from build123d import *

# Parameters (mm, degrees)
SKETCH1_W                = 70
SKETCH1_H                = 70
BOSS_EXTRUDE1_DEPTH      = 500
SKETCH2_W                = 250
SKETCH2_H                = 125
BOSS_EXTRUDE2_DEPTH      = 2
BOSS_EXTRUDE2_DEPTH_BACK = 40


with BuildPart() as part:
    # Sketch1 → Boss-Extrude1 (new body)
    with BuildSketch(Plane.XY):
        Rectangle(SKETCH1_W, SKETCH1_H)
    extrude(amount=BOSS_EXTRUDE1_DEPTH)

    # Sketch2 → Boss-Extrude2 (add, two sides)
    with BuildSketch(Plane(origin=(0, 35, 0), x_dir=(1, 0, 0), z_dir=(0, 1, 0))) as boss_extrude2_sk:
        with Locations((0, -437.5)):
            Rectangle(SKETCH2_W, SKETCH2_H)
    extrude(amount=BOSS_EXTRUDE2_DEPTH)
    extrude(boss_extrude2_sk.sketch, amount=-BOSS_EXTRUDE2_DEPTH_BACK)


solid = part.part
CAD build for the part. Positions are in the model's coordinates, mm. A direction names the side the tool comes from. Coordinates: 2 decimals unless noted, no trailing zeros. Order: outer loops, then holes, each group sorted by start corner. A loop starts at its lowest first (then second) coordinate and runs counter-clockwise, first axis right, second up. Notation, with made-up numbers: (49.5, 7) -> (79.5, 7) arc R18 ccw to (79.5, 21) -> close; hole circle Ø5 at (-19, 72.25). An arc over 180 degrees is marked (long way). Answer in a Markdown table with one row per item.
1) Drill centre lines: line 1 (X direction, y = -25, z = 326); line 2 (Z direction, x = -48.5, y = -1.5); line 3 (Y direction, x = -40.5, z = 452). Where is each one in solid material? Low to high.
Check values:
| item | result |
|---|---|
| line 1 | -35 to 35 |
| line 2 | 375 to 500 |
| line 3 | -5 to 37 |
2) Band-saw the part on A-A (y = 24). List the corners of the cut face in (x, z).
Check values:
| item | result |
|---|---|
| outline | (-125, 375) -> (-35, 375) -> (-35, 0) -> (35, 0) -> (35, 375) -> (125, 375) -> (125, 500) -> (-125, 500) -> close |
3) Flat gauge pins, fed straight in: P1, Ø6, axis at y = -16, z = 415, coming from the +X side; P2, Ø21, axis at y = 10.5, z = 317.5, coming from the -X side; P3, Ø2, axis at x = 52, y = 23, coming from the -Z side. Where does each tip first touch, or does it go through?
Check values:
| item | result |
|---|---|
| P1 | x = 35 |
| P2 | x = -35 |
| P3 | z = 375 |
4) Band-saw the part on B-B (z = 416). List the corners of the cut face in (x, y), and give its area (3 significant figures).
Check values:
| item | result |
|---|---|
| outline | (-125, -5) -> (-35, -5) -> (-35, -35) -> (35, -35) -> (35, -5) -> (125, -5) -> (125, 37) -> (-125, 37) -> close |
| area | 12,600 mm2 |
5) Band-saw the part on C-C (x = 24.5). List the corners of the cut face in (y, z).
Check values:
| item | result |
|---|---|
| outline | (-35, 0) -> (35, 0) -> (35, 375) -> (37, 375) -> (37, 500) -> (-35, 500) -> close |
6) Which spindle directions (+Z, -Z, +X, -X, +Y, -Y) get a long thin tool onto all of the face, cutting with end or side? Do faces 1 (the face through (0, 35, 185)), 2 (the face through (-81, -5, 437)), 3 (the face through (79, -5, 437)). Say none if no direction does.
Check values:
| item | result |
|---|---|
| face 1 | -Z, +X, -X, +Y |
| face 2 | +Z, -Z, -X, -Y |
| face 3 | +Z, -Z, +X, -Y |
7) Band-saw the part on D-D (y = -27). List the corners of the cut face in (x, z).
Check values:
| item | result |
|---|---|
| outline | (-35, 0) -> (35, 0) -> (35, 500) -> (-35, 500) -> close |
